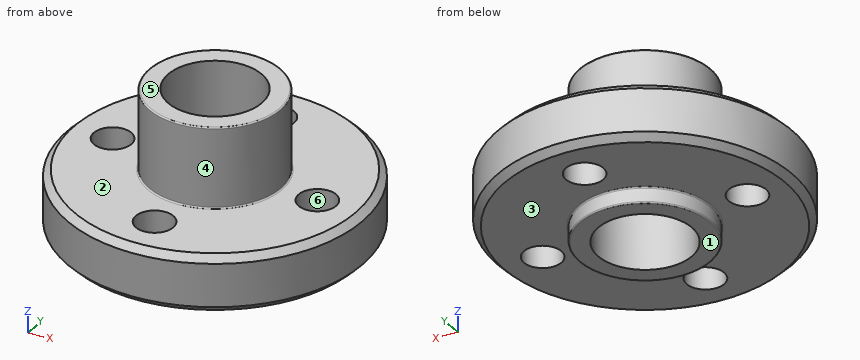
```python
from build123d import *

# Parameters (mm, degrees)
F0_R          = 11
F0_R_2        = 1.4
F0_R_3        = 4.9
F0_R_4        = 3.5
F1_DEPTH      = 4.22
F2_DEPTH      = 5.4
F2_DEPTH_BACK = 6
F3_SIZE       = 0.5
F4_R          = 0.1


with BuildPart() as f1:
    # F0 (on Top) → F1 (new body)
    with BuildSketch(Plane.XY):
        Circle(F0_R)
        with Locations((0, -7.6)):
            Circle(F0_R_2, mode=Mode.SUBTRACT)
        with Locations((-7.6, 0)):
            Circle(F0_R_2, mode=Mode.SUBTRACT)
        Circle(F0_R_3, mode=Mode.SUBTRACT)
        with Locations((7.6, 0)):
            Circle(F0_R_2, mode=Mode.SUBTRACT)
        with Locations((0, 7.6)):
            Circle(F0_R_2, mode=Mode.SUBTRACT)
        Circle(F0_R_3)
        Circle(F0_R_4, mode=Mode.SUBTRACT)
    extrude(amount=-F1_DEPTH)

    # F0 (on Top) → F2 (join, two sides)
    with BuildSketch(Plane.XY) as f2_sk:
        Circle(F0_R_3)
        Circle(F0_R_4, mode=Mode.SUBTRACT)
    extrude(amount=-F2_DEPTH)
    extrude(f2_sk.sketch, amount=F2_DEPTH_BACK)

    # F3
    f3_edges = [f1.edges().sort_by_distance(p)[0] for p in [
        (-11, 0, 0),
        (-11, 0, -4.22),
    ]]
    chamfer(f3_edges, length=F3_SIZE)

    # F4
    f4_edges = [f1.edges().sort_by_distance(p)[0] for p in [
        (-4.9, 0, 0),
        (-4.9, 0, 6),
        (-4.9, 0, -4.22),
        (-4.9, 0, -5.4),
    ]]
    fillet(f4_edges, radius=F4_R)


solid = f1.part
```
Can you work these out from the model? Positions are in its coordinate system, mm. Face numbers are marked on the shaded views. A direction names the side the tool comes from. Coordinates: 2 decimals unless noted, no trailing zeros. Loops run counter-clockwise (first coordinate to the right, second up) from the corner with the lowest first, then second, coordinate; pieces in that order, holes last. Notation, with made-up numbers: (76, 85) -> (99, 85) arc R19 ccw to (99, 104) -> close; hole circle Ø9 at (67, 36.5). An arc over 180 degrees is marked (long way). Answer as a JSON object with one key per item and string values.
1) For P1, Ø3, axis at x = 0, y = 7.6, coming from the +Z side; P2, Ø6, axis at x = -7, y = -7, coming from the -Z side; P3, Ø5.5, axis at x = 0, y = 0, coming from the -Z side; P4, Ø5, axis at y = 0, z = 0, coming from the -X side, each with a flat end and sliding along its axis, tell me the tip position at first contact or that it passes through.
Results:
{"P1": "stops at z = 0", "P2": "stops at z = -4.22", "P3": "passes through", "P4": "stops at x = -11"}
2) Thinking about a two-plate mould opening in X: for the marked faces 4, 5 and 6, which applies, pulls with the +X half, pulls with the -X half, needs draft (parallel to the pull), parting line crosses it, or undercut?
Results:
{"face 4": "parting line crosses it", "face 5": "needs draft", "face 6": "undercut"}
3) For the marked faces 1, 2 and 3, which set-ups out of +Z, -Z, +X, -X, +Y, -Y let a thin tool reach every point of the face, with its end or its side?
Results:
{"face 1": "-Z, +X, -X, +Y, -Y", "face 2": "+Z", "face 3": "-Z"}
4) Imagine slicing it at C-C (z = -1). Please give me the cut outline in (x, y), then the cut area to 3 significant figures.
Results:
{"outline": "circle Ø22 at (0, 0); hole circle Ø2.8 at (-7.6, 0); hole circle Ø7 at (0, 0); hole circle Ø2.8 at (0, -7.6); hole circle Ø2.8 at (0, 7.6); hole circle Ø2.8 at (7.6, 0)", "area": "317 mm^2"}
5) Imagine slicing it at B-B (x = 0). Count the separate pieces of the cut face and the enclosed holes in it, then the cut area to 3 significant figures.
Results:
{"separate pieces": "4", "enclosed holes": "0", "area": "59.3 mm^2"}
6) Imagine slicing it at A-A (z = 4.25). Please give me the cut outline in (x, y), then the cut area to 3 significant figures.
Results:
{"outline": "circle Ø9.8 at (0, 0); hole circle Ø7 at (0, 0)", "area": "36.9 mm^2"}
7) If I drill on line 1 (Y direction, x = 0, z = -3.15); line 2 (Y direction, x = 0, z = 4.25); line 3 (Z direction, x = 2.75, y = -8.5), over which ranges is the centre line in solid material (lowest first)?
Results:
{"line 1": "y = -11 to -9, -6.2 to -3.5, 3.5 to 6.2, 9 to 11", "line 2": "y = -4.9 to -3.5, 3.5 to 4.9", "line 3": "z = -4.22 to 0"}
